Source: CAD feature listing. Evaluate the final solid. Frame: model axes, mm. A direction names the side the tool comes from. Round coordinates to 2 decimals unless told otherwise and drop trailing zeros. Order: outer loops, then holes, each group sorted by start corner. A loop starts at its lowest first (then second) coordinate and runs counter-clockwise, first axis right, second up. Notation, with made-up numbers: (-19.5, 43.5) - (25.5, 43.5) arc R33 ccw to (25.5, 74.5) - close; hole circle Ø3 at (21.25, -22.5). An arc over 180 degrees is marked (long way). Use one line per item in the form item = value. Start each with the question number.
Q1. Ray query, line 1 (Y direction, x = 15.5, z = 1.5); line 2 (X direction, y = 9, z = 2.85); line 3 (X direction, y = -5, z = 3.75). Return the intervals inside material, ascending. Write a range as [from, to].
Q2. Cut plane D-D, the plane y = 2. Return the cut outline in (x, z), and give its area (3 significant figures).
Q3. Cut plane C-C, the plane x = -11.5. Return the cut outline in (y, z), and give its area (3 significant figures).
Q4. Pin query (flat end, axial travel): pin 1 Ø12 at (x, y) = (0, 4) entering from +Z; pin 2 Ø1.5 at (y, z) = (-18, 3) entering from +X. Return the tip coordinate at first contact, or that it passes through.
Q5. Draft query along X for faces 3 (the flat face through (-5, -4, 0)), 4 (the flat face through (18.85, -18.9, 2.76)), 5 (the flat face through (0, -20.1, 5)). Return one class per face: released by +X, released by -X, zero draft, split by the parting line, or undercut.
Q6. Cut plane B-B, the plane x = 0. Return the cut outline in (y, z), and give its area (3 significant figures).
Q7. Set-up query: faces 1 (the flat face through (18.9, 18.85, 2.76)), 2 (the flat face through (-19.4, 0.1, 4)). Return all of +Z, -Z, +X, -X, +Y, -Y with unobstructed straight access to the full face (end or side cutting, diameter ignored); none if empty.
Q8. Cut plane A-A, the plane z = 5.1. Return the cut outline in (x, y), and give its area (3 significant figures).
from build123d import *

# Parameters (mm, degrees)
SKETCH_1_R      = 5
SKETCH_1_R_2    = 1.6
EXTRUDE_3_DEPTH = 1
SKETCH_3_R      = 1.6
EXTRUDE_4_DEPTH = 3
EXTRUDE_5_DEPTH = 1.6


with BuildPart() as part:
    # 草图1 → 凸台-拉伸3 (new body)
    with BuildSketch(Plane.XY):
        Polygon((-21, 16.75), (-21, -16.75), (-16.75, -21), (16.75, -21), (21, -16.75), (21, 16.75), (16.75, 21), (-16.75, 21), align=None)
        Circle(SKETCH_1_R, mode=Mode.SUBTRACT)
        with Locations((-15.5, 15.5)):
            Circle(SKETCH_1_R_2, mode=Mode.SUBTRACT)
        with Locations((15.5, 15.5)):
            Circle(SKETCH_1_R_2, mode=Mode.SUBTRACT)
        with Locations((-15.5, -15.5)):
            Circle(SKETCH_1_R_2, mode=Mode.SUBTRACT)
        with Locations((15.5, -15.5)):
            Circle(SKETCH_1_R_2, mode=Mode.SUBTRACT)
        with BuildLine():
            Line((13, 6), (13, 0))
            ThreePointArc((13, 0), (14.025126266, -2.474873734), (16.5, -3.5))
            Line((16.5, -3.5), (20, -3.5))
            Line((20, -3.5), (20, 9.5))
            Line((20, 9.5), (16.5, 9.5))
            ThreePointArc((16.5, 9.5), (14.025126266, 8.474873734), (13, 6))
        make_face(mode=Mode.SUBTRACT)
    extrude(amount=EXTRUDE_3_DEPTH)

    # 草图3 → 凸台-拉伸4 (add)
    with BuildSketch(Plane.XY.offset(1)):
        Polygon((-16.75, 21), (-21, 16.75), (-21, -16.75), (-16.75, -21), (16.75, -21), (21, -16.75), (21, 16.75), (16.75, 21), align=None)
        with Locations((-15.5, 15.5)):
            Circle(SKETCH_3_R, mode=Mode.SUBTRACT)
        with Locations((15.5, 15.5)):
            Circle(SKETCH_3_R, mode=Mode.SUBTRACT)
        with Locations((-15.5, -15.5)):
            Circle(SKETCH_3_R, mode=Mode.SUBTRACT)
        with Locations((15.5, -15.5)):
            Circle(SKETCH_3_R, mode=Mode.SUBTRACT)
        with BuildLine():
            Line((-12.5, 15.5), (-12.5, 19.5))
            Line((-12.5, 19.5), (12.5, 19.5))
            Line((12.5, 19.5), (12.5, 15.5))
            ThreePointArc((12.5, 15.5), (13.378679656, 13.378679656), (15.5, 12.5))
            Line((15.5, 12.5), (19, 12.5))
            Line((19, 12.5), (19, 9.5))
            Line((19, 9.5), (20, 9.5))
            Line((20, 9.5), (20, -3.5))
            Line((20, -3.5), (19, -3.5))
            Line((19, -3.5), (19, -12.5))
            Line((19, -12.5), (15.5, -12.5))
            ThreePointArc((15.5, -12.5), (13.378679656, -13.378679656), (12.5, -15.5))
            Line((12.5, -15.5), (12.5, -19.5))
            Line((12.5, -19.5), (-12.5, -19.5))
            Line((-12.5, -19.5), (-12.5, -15.5))
            ThreePointArc((-12.5, -15.5), (-13.378679656, -13.378679656), (-15.5, -12.5))
            Line((-15.5, -12.5), (-19, -12.5))
            Line((-19, -12.5), (-19, 12.5))
            Line((-19, 12.5), (-15.5, 12.5))
            ThreePointArc((-15.5, 12.5), (-13.378679656, 13.378679656), (-12.5, 15.5))
        make_face(mode=Mode.SUBTRACT)
    extrude(amount=EXTRUDE_4_DEPTH)

    # 草图4 → 凸台-拉伸5 (add)
    with BuildSketch(Plane.XY.offset(4)):
        Polygon((-16.75, 21), (-21, 16.75), (-21, -16.75), (-16.75, -21), (16.75, -21), (21, -16.75), (21, 16.75), (16.75, 21), align=None)
        with BuildLine():
            Line((-20.1, 13), (-20.1, -13))
            ThreePointArc((-20.1, -13), (-18.020458146, -18.020458146), (-13, -20.1))
            Line((-13, -20.1), (13, -20.1))
            ThreePointArc((13, -20.1), (18.020458146, -18.020458146), (20.1, -13))
            Line((20.1, -13), (20.1, 13))
            ThreePointArc((20.1, 13), (18.020458146, 18.020458146), (13, 20.1))
            Line((13, 20.1), (-13, 20.1))
            ThreePointArc((-13, 20.1), (-18.020458146, 18.020458146), (-20.1, 13))
        make_face(mode=Mode.SUBTRACT)
    extrude(amount=EXTRUDE_5_DEPTH)


solid = part.part
Completed:
q1.line_1 = [-21, -17.1], [-13.9, -12.5], [12.5, 13.9], [17.1, 21]
q1.line_2 = [-21, -19], [20, 21]
q1.line_3 = [-21, -19], [19, 21]
q2.outline = (-21, 0) - (-4.58, 0) - (-4.58, 1) - (-19, 1) - (-19, 4) - (-20.1, 4) - (-20.1, 5.6) - (-21, 5.6) - close; (4.58, 0) - (13, 0) - (13, 1) - (4.58, 1) - close; (20, 0) - (21, 0) - (21, 5.6) - (20.1, 5.6) - (20.1, 4) - (20, 4) - close
q2.area = 37.7 mm2
q3.outline = (-21, 0) - (21, 0) - (21, 5.6) - (20.1, 5.6) - (20.1, 4) - (19.5, 4) - (19.5, 1) - (-19.5, 1) - (-19.5, 4) - (-20.1, 4) - (-20.1, 5.6) - (-21, 5.6) - close
q3.area = 53.9 mm2
q4.pin_1 = 1
q4.pin_2 = 20.5
q5.face_3 = zero draft
q5.face_4 = released by +X
q5.face_5 = undercut
q6.outline = (-21, 0) - (-5, 0) - (-5, 1) - (-19.5, 1) - (-19.5, 4) - (-20.1, 4) - (-20.1, 5.6) - (-21, 5.6) - close; (5, 0) - (21, 0) - (21, 5.6) - (20.1, 5.6) - (20.1, 4) - (19.5, 4) - (19.5, 1) - (5, 1) - close
q6.area = 43.9 mm2
q7.face_1 = +Z, -Z, +X, +Y
q7.face_2 = +Z
q8.outline = (-21, -16.75) - (-16.75, -21) - (16.75, -21) - (21, -16.75) - (21, 16.75) - (16.75, 21) - (-16.75, 21) - (-21, 16.75) - close; hole (-20.1, -13) arc R7.1 ccw to (-13, -20.1) - (13, -20.1) arc R7.1 ccw to (20.1, -13) - (20.1, 13) arc R7.1 ccw to (13, 20.1) - (-13, 20.1) arc R7.1 ccw to (-20.1, 13) - close
q8.area = 155 mm2
